Can you work these out from the model? Positions are in its coordinate system, mm. Face numbers are marked on the shaded views. Give positions to 0.01 mm unless a question says otherwise; leave off trailing zeros. Loops run counter-clockwise (first coordinate to the right, second up) from the corner with the lowest first, then second, coordinate; pieces in that order, holes last. Notation, with made-up numbers: (4.25, -2) -> (52.25, -2) arc R26 ccw to (52.25, 36) -> close; hole circle Ø6 at (75, 62.25). An arc over 180 degrees is marked (long way). Return JSON: item names as keys, results as strings. Group by question number.
Q1. Suppose I cut it at B-B, the plane x = 0. Please give me the cut outline in (y, z).
Q2. Suppose I cut it at A-A, the plane z = 1.5. Please give me the cut outline in (x, y), and give its area (3 significant figures).
Q3. Suppose I cut it at D-D, the plane y = -10. Please give me the cut outline in (x, z).
Q4. I need wall thicknesses on line 1 along X through (y, z) = (-1.5, 0); line 2 along Y through (x, z) = (-50.5, 0); line 3 along X through (y, z) = (-16.45, -10). Which ranges of each line are inside material? Lowest first, please. Write a range as [from, to].
Q5. Suppose I cut it at C-C, the plane z = -10. Please give me the cut outline in (x, y).
Q6. Will these pins go through, and if not, where does the flat tip stop? pin 1 (11 mm diameter, centred on x = -1.5, z = -9.5, fed in from -Y); pin 2 (6 mm diameter, centred on x = -16.5, y = -11, fed in from -Z); pin 3 (2.5 mm diameter, centred on y = -16.5, z = -12, fed in from +X); pin 4 (1.5 mm diameter, centred on y = -17.5, z = -9.5, fed in from -X).
Q7. Thinking about a two-plate mould opening in X: for the marked faces 1, 2 and 3, which applies, pulls with the +X half, pulls with the -X half, needs draft (parallel to the pull), parting line crosses it, or undercut?
```python
from build123d import *

# Parameters (mm, degrees)
SKETCH1_W           = 100
SKETCH1_H           = 10
SKETCH1_R           = 2.5
SKETCH1_W_2         = 10
BOSS_EXTRUDE1_DEPTH = 20
SKETCH2_W           = 10
SKETCH2_H           = 10
CUT_EXTRUDE1_DEPTH  = 10
SKETCH5_W           = 10
SKETCH5_H           = 10
CUT_EXTRUDE4_DEPTH  = 10
CUT_EXTRUDE3_REACH  = 66.031
SKETCH4_R           = 5


with BuildPart() as part:
    # Sketch1 → Boss-Extrude1 (new body)
    # profile 1 of 2: a face of its own
    with BuildSketch(Plane(origin=(0, 0, 0), x_dir=(1, 0, 0), z_dir=(0, 1, 0))):
        with Locations((-10, 0)):
            Rectangle(SKETCH1_W, SKETCH1_H)
        with Locations(Location((-55, 0, 0), (0, 0, 270))):
            Circle(SKETCH1_R, mode=Mode.SUBTRACT)
    # profile 2 of 2: a face of its own
    with BuildSketch(Plane(origin=(0, 0, 0), x_dir=(1, 0, 0), z_dir=(0, 1, 0))):
        with Locations((0, 10)):
            Rectangle(SKETCH1_W_2, SKETCH1_H)
        with Locations(Location((0, 10, 0), (0, 0, 270))):
            Circle(SKETCH1_R, mode=Mode.SUBTRACT)
    extrude(amount=-BOSS_EXTRUDE1_DEPTH)

    # Sketch2 → Cut-Extrude1 (cut)
    with BuildSketch(Plane.ZY.offset(60)):
        with Locations((0, -10)):
            Rectangle(SKETCH2_W, SKETCH2_H)
    extrude(amount=-CUT_EXTRUDE1_DEPTH, mode=Mode.SUBTRACT)

    # Sketch5 → Cut-Extrude4 (cut)
    with BuildSketch(Plane(origin=(0, 0, -15), x_dir=(-1, 0, 0), z_dir=(0, 0, -1))):
        with Locations((0, -10)):
            Rectangle(SKETCH5_W, SKETCH5_H)
    extrude(amount=-CUT_EXTRUDE4_DEPTH, mode=Mode.SUBTRACT)

    # Sketch4 → Cut-Extrude3 (cut, up to next)
    with BuildSketch(Plane(origin=(0, 0, -5), x_dir=(-1, 0, 0), z_dir=(0, 0, -1)), mode=Mode.PRIVATE) as cut_extrude3_sk1:
        with Locations((-30, -10)):
            Circle(SKETCH4_R)
    cut_extrude3_tool1 = extrude(cut_extrude3_sk1.sketch, amount=-CUT_EXTRUDE3_REACH, mode=Mode.PRIVATE) & part.part
    add(cut_extrude3_tool1.solids().sort_by_distance((30, -10, -5))[0], mode=Mode.SUBTRACT)


solid = part.part
```
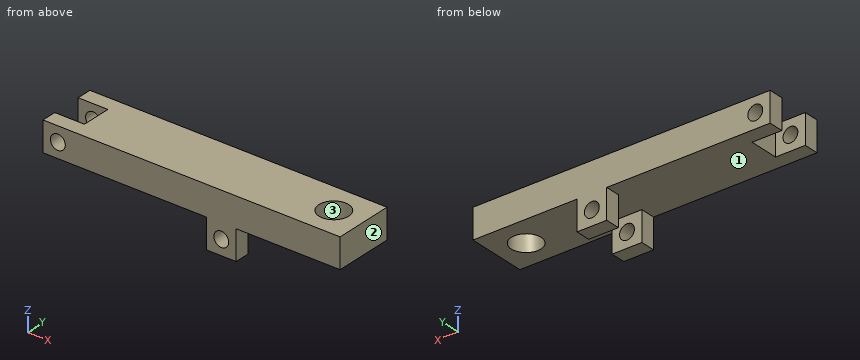
Ans:
{
 "1": {"outline": "(-20, -15) -> (-15, -15) -> (-15, -12.5) -> (-20, -12.5) -> close; (-20, -7.5) -> (-15, -7.5) -> (-15, -5) -> (-5, -5) -> (-5, -7.5) -> (0, -7.5) -> (0, 5) -> (-20, 5) -> close; (-5, -15) -> (0, -15) -> (0, -12.5) -> (-5, -12.5) -> close"},
 "2": {"outline": "(-60, -20) -> (-57, -20) -> (-57, -15) -> (-60, -15) -> close; (-60, -5) -> (-57, -5) -> (-57, 0) -> (-60, 0) -> close; (-53, -20) -> (40, -20) -> (40, 0) -> (-53, 0) -> (-53, -5) -> (-50, -5) -> (-50, -15) -> (-53, -15) -> close; hole circle Ø10 at (30, -10)", "area": "1,780 mm^2"},
 "3": {"outline": "(-50, -5) -> (25, -5) -> (25, 5) -> (-50, 5) -> close; (35, -5) -> (40, -5) -> (40, 5) -> (35, 5) -> close"},
 "4": {"line 1": "x = [-60, -57.5], [-52.5, 40]", "line 2": "y = [-20, -15], [-5, 0]", "line 3": "x = [-5, -2.5], [2.5, 5]"},
 "5": {"outline": "(-5, -20) -> (-2.5, -20) -> (-2.5, -15) -> (-5, -15) -> close; (-5, -5) -> (-2.5, -5) -> (-2.5, 0) -> (-5, 0) -> close; (2.5, -20) -> (5, -20) -> (5, -15) -> (2.5, -15) -> close; (2.5, -5) -> (5, -5) -> (5, 0) -> (2.5, 0) -> close"},
 "6": {"pin 1": "stops at y = -20", "pin 2": "stops at z = -5", "pin 3": "stops at x = 5", "pin 4": "stops at x = -5"},
 "7": {"face 1": "needs draft", "face 2": "pulls with the +X half", "face 3": "undercut"}
}
